Here's the drawing with two shaded views (mm, measured from the low corner). I have some questions. A direction names the side the tool comes from. Round coordinates to 2 decimals unless told otherwise and drop trailing zeros. Write each loop counter-clockwise with the first axis right and the second up, starting at its lowest first coordinate (ties: lowest second). Pieces come first, ordered by that corner, then holes. Notation, with made-up numbers: M -39,-17.5 L 12,-17.5 A18 ccw 12,1.5 Z; hole C 79,80 d2. An arc over 180 degrees is marked long. Answer as a JSON object with one key per item and string values. Group by question number.
1) Please list where these lines run through material, in increasing order: L1, parallel to Y at x = 22, z = 133 (3 decimals); L2, parallel to X at y = 2.5, z = 127; L3, parallel to X at y = 9.5, z = 119.5 (3 decimals). Write a range as [from, to].
2) Suppose I cut it at C-C, the plane x = 6. Write out the boundary of the cut face in (y, z) (3 decimals).
3) I'm going to push a flat-ended pin straight in: pin 1 Ø8.5 at (x, z) = (25.4, 127) entering from -Y. Where does the tip first touch, or does it pass through?
4) Suppose I cut it at B-B, the plane x = 25.4. Write out the boundary of the cut face in (y, z) (3 decimals).
5) If we mould it in two halves opening along X, with no side actions, what happens to the marked faces 1, 2 and 3? For each: +X half, -X half, draft (parallel to the pull), parting line (faces both ways), or undercut.
6) On a 3-axis mill with a long thin cutter (end or side, diameter ignored), from which of +Z, -Z, +X, -X, +Y, -Y can I reach the whole of each face in a straight line? I mean the marked faces 4 and 5. Say none if no direction works.
7) Suppose I cut it at A-A, the plane z = 127. Write out the boundary of the cut face in (x, y) (3 decimals), and give its area (3 significant figures).
8) Suppose I cut it at D-D, the plane y = 20.75. Write out the boundary of the cut face in (x, z) (3 decimals).
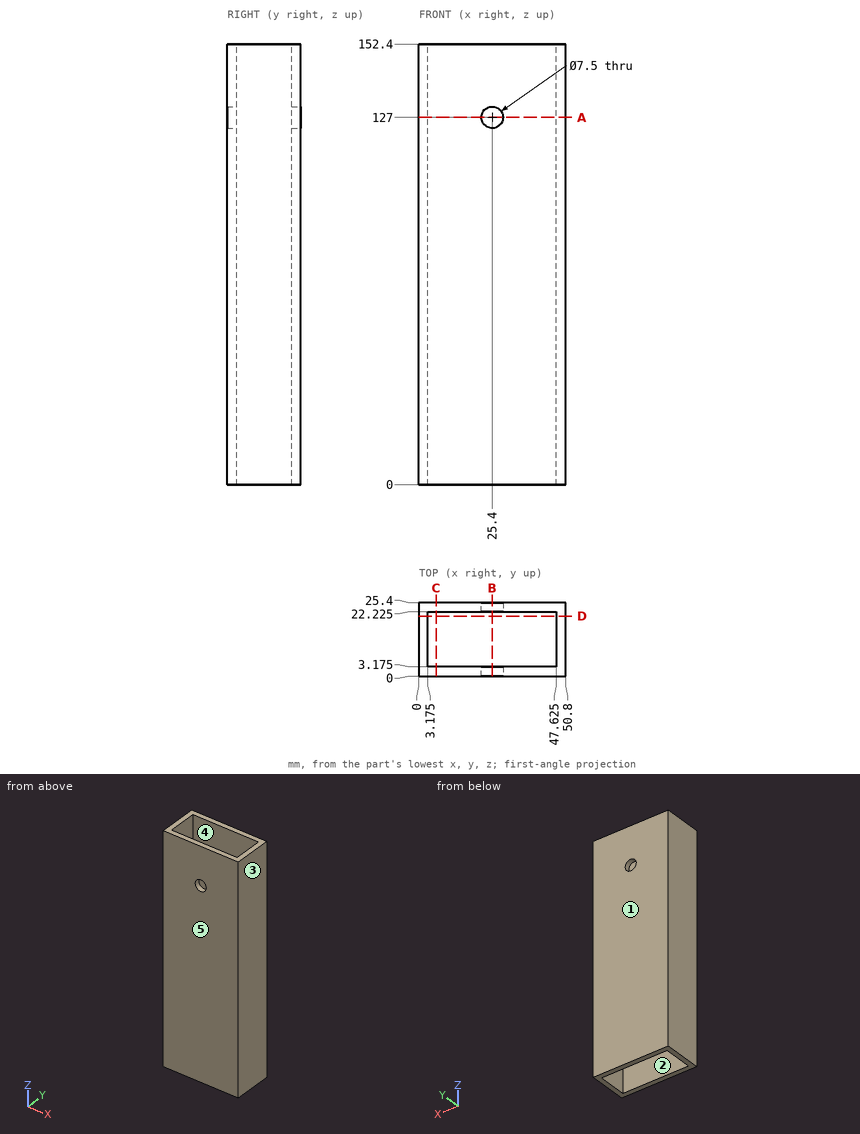
Results:
{
 "1": {"L1": "[0, 3.175], [22.225, 25.4]", "L2": "[0, 21.65], [29.15, 50.8]", "L3": "[0, 3.175], [47.625, 50.8]"},
 "2": {"outline": "M 0,0 L 3.175,0 L 3.175,152.4 L 0,152.4 Z; M 22.225,0 L 25.4,0 L 25.4,152.4 L 22.225,152.4 Z"},
 "3": {"pin 1": "y = 0"},
 "4": {"outline": "M 0,0 L 3.175,0 L 3.175,123.25 L 0,123.25 Z; M 0,130.75 L 3.175,130.75 L 3.175,152.4 L 0,152.4 Z; M 22.225,0 L 25.4,0 L 25.4,123.25 L 22.225,123.25 Z; M 22.225,130.75 L 25.4,130.75 L 25.4,152.4 L 22.225,152.4 Z"},
 "5": {"face 1": "draft", "face 2": "undercut", "face 3": "+X half"},
 "6": {"face 4": "+Z, -Z", "face 5": "+Z, -Z, +X, -X, -Y"},
 "7": {"outline": "M 0,0 L 21.65,0 L 21.65,3.175 L 3.175,3.175 L 3.175,22.225 L 21.65,22.225 L 21.65,25.4 L 0,25.4 Z; M 29.15,0 L 50.8,0 L 50.8,25.4 L 29.15,25.4 L 29.15,22.225 L 47.625,22.225 L 47.625,3.175 L 29.15,3.175 Z", "area": "396 mm^2"},
 "8": {"outline": "M 0,0 L 3.175,0 L 3.175,152.4 L 0,152.4 Z; M 47.625,0 L 50.8,0 L 50.8,152.4 L 47.625,152.4 Z"}
}
